For this review, take the finished solid that the model builds, in its own axes (mm). Face numbers are marked on the shaded views. Give positions to 0.01 mm unless a question says otherwise; leave off trailing zeros. Order: outer loops, then holes, each group sorted by start corner. A loop starts at its lowest first (then second) coordinate and runs counter-clockwise, first axis right, second up. Notation, with made-up numbers: (-1.75, 48) - (44.25, 48) arc R13 cw to (44.25, 69) - close; hole circle Ø7 at (86, 8). An arc over 180 degrees is marked (long way). Answer as a JSON object with one key per item and string values. Group by question number.
from build123d import *

# Parameters (mm, degrees)
BOSS_EXTRU_5_DEPTH = 25
ESQUISSE7_R        = 8
ESQUISSE7_R_2      = 7.5
BOSS_EXTRU_7_DEPTH = 5
BOSS_EXTRU_6_DEPTH = 10


# Read off the part's stored shape, not the designer's step: Boss.-Extru.5
with BuildPart() as part:
    # Boss.-Extru.5 outline → Boss.-Extru.5 (new body)
    # profile 1 of 2: a face of its own
    with BuildSketch(Plane.XY):
        with BuildLine():
            Line((-8.5, -13.5), (8.5, -13.5))
            ThreePointArc((8.5, -13.5), (12.035533906, -12.035533906), (13.5, -8.5))
            Line((13.5, -8.5), (13.5, 8.5))
            ThreePointArc((13.5, 8.5), (12.035533906, 12.035533906), (8.5, 13.5))
            Line((8.5, 13.5), (-8.5, 13.5))
            ThreePointArc((-8.5, 13.5), (-12.035533906, 12.035533906), (-13.5, 8.5))
            Line((-13.5, 8.5), (-13.5, -8.5))
            ThreePointArc((-13.5, -8.5), (-12.035533906, -12.035533906), (-8.5, -13.5))
        make_face()
        with BuildLine():
            Line((-10, 3.5), (-10, 8.5))
            ThreePointArc((-10, 8.5), (-9.560660172, 9.560660172), (-8.5, 10))
            Line((-8.5, 10), (-3.5, 10))
            Line((-3.5, 10), (-3.5, 9.5))
            Line((-3.5, 9.5), (-3, 9.5))
            Line((-3, 9.5), (-3, 8.5))
            Line((-3, 8.5), (-6, 8.5))
            Line((-6, 8.5), (-6, 7.060660172))
            Line((-6, 7.060660172), (-3.439339828, 4.5))
            Line((-3.439339828, 4.5), (-0.866025404, 4.5))
            Line((-0.866025404, 4.5), (0, 4))
            Line((0, 4), (0.866025404, 4.5))
            Line((0.866025404, 4.5), (3.439339828, 4.5))
            Line((3.439339828, 4.5), (6, 7.060660172))
            Line((6, 7.060660172), (6, 8.5))
            Line((6, 8.5), (3, 8.5))
            Line((3, 8.5), (3, 9.5))
            Line((3, 9.5), (3.5, 9.5))
            Line((3.5, 9.5), (3.5, 10))
            Line((3.5, 10), (8.5, 10))
            ThreePointArc((8.5, 10), (9.560660172, 9.560660172), (10, 8.5))
            Line((10, 8.5), (10, 3.5))
            Line((10, 3.5), (9.5, 3.5))
            Line((9.5, 3.5), (9.5, 3))
            Line((9.5, 3), (8.5, 3))
            Line((8.5, 3), (8.5, 6))
            Line((8.5, 6), (7.060660172, 6))
            Line((7.060660172, 6), (4.5, 3.439339828))
            Line((4.5, 3.439339828), (4.5, 0.866025404))
            Line((4.5, 0.866025404), (4, 0))
            Line((4, 0), (4.5, -0.866025404))
            Line((4.5, -0.866025404), (4.5, -3.439339828))
            Line((4.5, -3.439339828), (7.060660172, -6))
            Line((7.060660172, -6), (8.5, -6))
            Line((8.5, -6), (8.5, -3))
            Line((8.5, -3), (9.5, -3))
            Line((9.5, -3), (9.5, -3.5))
            Line((9.5, -3.5), (10, -3.5))
            Line((10, -3.5), (10, -8.5))
            ThreePointArc((10, -8.5), (9.560660172, -9.560660172), (8.5, -10))
            Line((8.5, -10), (3.5, -10))
            Line((3.5, -10), (3.5, -9.5))
            Line((3.5, -9.5), (3, -9.5))
            Line((3, -9.5), (3, -8.5))
            Line((3, -8.5), (6, -8.5))
            Line((6, -8.5), (6, -7.060660172))
            Line((6, -7.060660172), (3.439339828, -4.5))
            Line((3.439339828, -4.5), (0.866025404, -4.5))
            Line((0.866025404, -4.5), (0, -4))
            Line((0, -4), (-0.866025404, -4.5))
            Line((-0.866025404, -4.5), (-3.439339828, -4.5))
            Line((-3.439339828, -4.5), (-6, -7.060660172))
            Line((-6, -7.060660172), (-6, -8.5))
            Line((-6, -8.5), (-3, -8.5))
            Line((-3, -8.5), (-3, -9.5))
            Line((-3, -9.5), (-3.5, -9.5))
            Line((-3.5, -9.5), (-3.5, -10))
            Line((-3.5, -10), (-8.5, -10))
            ThreePointArc((-8.5, -10), (-9.560660172, -9.560660172), (-10, -8.5))
            Line((-10, -8.5), (-10, -3.5))
            Line((-10, -3.5), (-9.5, -3.5))
            Line((-9.5, -3.5), (-9.5, -3))
            Line((-9.5, -3), (-8.5, -3))
            Line((-8.5, -3), (-8.5, -6))
            Line((-8.5, -6), (-7.060660172, -6))
            Line((-7.060660172, -6), (-4.5, -3.439339828))
            Line((-4.5, -3.439339828), (-4.5, -0.866025404))
            Line((-4.5, -0.866025404), (-4, 0))
            Line((-4, 0), (-4.5, 0.866025404))
            Line((-4.5, 0.866025404), (-4.5, 3.439339828))
            Line((-4.5, 3.439339828), (-7.060660172, 6))
            Line((-7.060660172, 6), (-8.5, 6))
            Line((-8.5, 6), (-8.5, 3))
            Line((-8.5, 3), (-9.5, 3))
            Line((-9.5, 3), (-9.5, 3.5))
            Line((-9.5, 3.5), (-10, 3.5))
        make_face(mode=Mode.SUBTRACT)
    # profile 2 of 2: a face of its own
    with BuildSketch(Plane.XY):
        with BuildLine():
            Line((1.949592103, 3.000876196), (1.276279893, 2.435900169))
            ThreePointArc((1.276279893, 2.435900169), (0.001756003, 2.749999439), (-1.273167982, 2.43752811))
            Line((-1.273167982, 2.43752811), (-1.947287092, 3.003181207))
            Line((-1.947287092, 3.003181207), (-3.000876196, 1.949592103))
            Line((-3.000876196, 1.949592103), (-2.435900169, 1.276279893))
            ThreePointArc((-2.435900169, 1.276279893), (-2.749999439, 0.001756003), (-2.43752811, -1.273167982))
            Line((-2.43752811, -1.273167982), (-3.003181207, -1.947287092))
            Line((-3.003181207, -1.947287092), (-1.949592103, -3.000876196))
            Line((-1.949592103, -3.000876196), (-1.276279893, -2.435900169))
            ThreePointArc((-1.276279893, -2.435900169), (-0.001756003, -2.749999439), (1.273167982, -2.43752811))
            Line((1.273167982, -2.43752811), (1.947287092, -3.003181207))
            Line((1.947287092, -3.003181207), (3.000876196, -1.949592103))
            Line((3.000876196, -1.949592103), (2.435900169, -1.276279893))
            ThreePointArc((2.435900169, -1.276279893), (2.749999439, -0.001756003), (2.43752811, 1.273167982))
            Line((2.43752811, 1.273167982), (3.003181207, 1.947287092))
            Line((3.003181207, 1.947287092), (1.949592103, 3.000876196))
        make_face()
    extrude(amount=BOSS_EXTRU_5_DEPTH)

    # Esquisse7 → Boss.-Extru.7 (add)
    with BuildSketch(Plane.ZY.offset(13.5)):
        with Locations(Location((12.5, 0, 0), (0, 0, 180))):
            Circle(ESQUISSE7_R)
        with Locations((12.5, 0)):
            Circle(ESQUISSE7_R_2, mode=Mode.SUBTRACT)
    extrude(amount=BOSS_EXTRU_7_DEPTH)

    # Esquisse6 → Boss.-Extru.6 (add)
    with BuildSketch(Plane.XY.offset(25)):
        with BuildLine():
            Line((-13.5, 8.5), (-13.5, -8.5))
            ThreePointArc((-13.5, -8.5), (-12.035533906, -12.035533906), (-8.5, -13.5))
            Line((-8.5, -13.5), (8.5, -13.5))
            ThreePointArc((8.5, -13.5), (12.035533906, -12.035533906), (13.5, -8.5))
            Line((13.5, -8.5), (13.5, 8.5))
            ThreePointArc((13.5, 8.5), (12.035533906, 12.035533906), (8.5, 13.5))
            Line((8.5, 13.5), (-8.5, 13.5))
            ThreePointArc((-8.5, 13.5), (-12.035533906, 12.035533906), (-13.5, 8.5))
        make_face()
    extrude(amount=BOSS_EXTRU_6_DEPTH)


solid = part.part
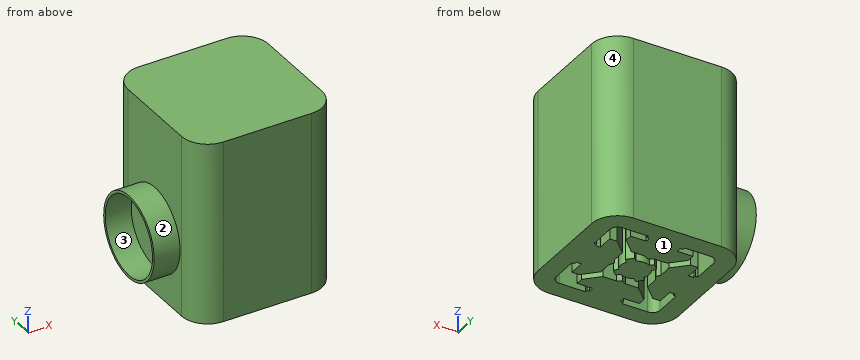
1) For line 1 (X direction, y = 0, z = 8); line 2 (X direction, y = -2.25, z = 13), list the stretches that pass through material, from the lowest coordinate up.
2) Consider section C-C (z = 26). Give the boundary of the cut face in (x, y), plus the area to 3 significant figures.
3) For pin 1 (1.1 mm diameter, centred on y = -9, z = 10, fed in from -X), flat-tipped, find the tip position at first contact; note if it passes through.
4) Consider section A-A (z = 12.5). Give the number of separate pieces and of enclosed holes in the cut face, plus the area to 3 significant figures.
5) Consider section D-D (x = -5). Give the boundary of the cut face in (y, z).
6) Consider section B-B (x = -14). Give the boundary of the cut face in (y, z).
7) Mouldability with a two-part tool opening along Z and no side actions: class the marked faces 1, 2, 3 and 4 as released by +Z, released by -Z, zero draft, split by the parting line, or undercut.
Result set:
{
 "1": {"line 1": "x = -13.5 to -4, -2.75 to 2.75, 4 to 13.5", "line 2": "x = -13.5 to -4.5, -2.7 to 2.7, 4.5 to 13.5"},
 "2": {"outline": "(-13.5, -8.5) arc R5 ccw to (-8.5, -13.5) - (8.5, -13.5) arc R5 ccw to (13.5, -8.5) - (13.5, 8.5) arc R5 ccw to (8.5, 13.5) - (-8.5, 13.5) arc R5 ccw to (-13.5, 8.5) - close", "area": "708 mm2"},
 "3": {"pin 1": "stops at x = -13.5"},
 "4": {"separate pieces": "2", "enclosed holes": "1", "area": "549 mm2"},
 "5": {"outline": "(-13.5, 0) - (-10, 0) - (-10, 25) - (-8.5, 25) - (-8.5, 0) - (-6.06, 0) - (-6.06, 25) - (-3.94, 25) - (-3.94, 0) - (3.94, 0) - (3.94, 25) - (6.06, 25) - (6.06, 0) - (8.5, 0) - (8.5, 25) - (10, 25) - (10, 0) - (13.5, 0) - (13.5, 35) - (-13.5, 35) - close"},
 "6": {"outline": "circle Ø16 at (0, 12.5); hole circle Ø15 at (0, 12.5)"},
 "7": {"face 1": "released by -Z", "face 2": "split by the parting line", "face 3": "undercut", "face 4": "zero draft"}
}
